from build123d import *

# Parameters (mm, degrees)
F0_W           = 9.5
F0_H           = 60
F1_DEPTH       = 4.5
F4_D           = 3.1
F4_CBORE_D     = 5.9
F4_CBORE_DEPTH = 2.2
F5_DEPTH       = 25
F6_SIZE        = 5
F7_R           = 3


with BuildPart() as f1:
    # F0 (on Top) → F1 (new body)
    with BuildSketch(Plane.XY):
        with Locations((4.75, 30)):
            Rectangle(F0_W, F0_H)
    extrude(amount=F1_DEPTH)

    # F4 (through all)
    with Locations(Plane.XY.offset(4.5)):
        with Locations((5.4, 36.5), (5.4, 5.5)):
            CounterBoreHole(F4_D / 2, F4_CBORE_D / 2, F4_CBORE_DEPTH)

    # F3 (on face) → F5 (cut)
    with BuildSketch(Plane.XY.offset(4.5)):
        with BuildLine():
            Line((6.25, 57.5), (3.25, 57.5))
            ThreePointArc((3.25, 57.5), (2.542893, 57.207107), (2.25, 56.5))
            Line((2.25, 56.5), (2.25, 44))
            ThreePointArc((2.25, 44), (2.542893, 43.292893), (3.25, 43))
            Line((3.25, 43), (6.25, 43))
            ThreePointArc((6.25, 43), (6.957107, 43.292893), (7.25, 44))
            Line((7.25, 44), (7.25, 56.5))
            ThreePointArc((7.25, 56.5), (6.957107, 57.207107), (6.25, 57.5))
        make_face()
    extrude(amount=-F5_DEPTH, mode=Mode.SUBTRACT)

    # F6
    f6_edges = [f1.edges().sort_by_distance(p)[0] for p in [
        (0, 0, 2.25),
    ]]
    chamfer(f6_edges, length=F6_SIZE)

    # F7
    f7_edges = [f1.edges().sort_by_distance(p)[0] for p in [
        (0, 60, 2.25),
        (9.5, 60, 2.25),
    ]]
    fillet(f7_edges, radius=F7_R)


solid = f1.part
Model file for the job. Use its own axes, mm. A direction names the side the tool comes from. Give positions to 0.01 mm unless a question says otherwise; leave off trailing zeros. Write each loop counter-clockwise with the first axis right and the second up, starting at its lowest first coordinate (ties: lowest second). Pieces come first, ordered by that corner, then holes. Notation, with made-up numbers: M 21,-27 L 33,-27 A5 ccw 33,-18 Z; hole C 50,-39 d11. An arc over 180 degrees is marked long. One line per item, written item: value. Start each with the question number.
Q1. Saw through at A-A, the plane z = 1. Write the cut outline in (x, y).
Q2. 3-axis set-ups, long thin cutter, end or side, ignore diameter. For faces 1 (the flat face through (5, 24, 0)), 2 (the flat face through (7, 4, 2.3)), 3 (the flat face through (5, 43, 2)): which of +Z, -Z, +X, -X, +Y, -Y reach the whole face in a straight line?
Q3. Probe probe 1 along Y at (x, z) = (5.4, 3.3); probe 2 along Y at (x, z) = (5.4, 1.4); probe 3 along Y at (x, z) = (7.5, 4.35). List the from-to ranges inside material, lowest first. Write a range as [from, to].
Q4. Drop flat-ended pins along their axis: pin 1 Ø3.5 at (x, y) = (5.4, 36.5) entering from +Z; pin 2 Ø2 at (x, z) = (8.5, 2) entering from +Y. Give the stop position or say it passes through.
Q5. Saw through at D-D, the plane y = 4.5. Write the cut outline in (x, z).
Q6. Saw through at C-C, the plane z = 3.9. Write the cut outline in (x, y).
Q7. Saw through at B-B, the plane y = 36.5. Write the cut outline in (x, z).
Q8. Two-plate mould, pull along X, no slides. Class faces 4 (the flat face through (5, 24, 4.5)), 5 (the cylindrical face through (6.949, 43.285, 2.282)), 6 (the cylindrical face through (2.535, 43.301, 2.282)), 7 (the cylindrical face through (8.6, 59.14, 2.28)): +X half, -X half, draft (parallel to the pull), parting line (faces both ways), or undercut.
Output values:
1. outline: M 0,5 L 5,0 L 9.5,0 L 9.5,57 A3 ccw 6.5,60 L 3,60 A3 ccw 0,57 Z; hole M 2.25,44 A1 ccw 3.25,43 L 6.25,43 A1 ccw 7.25,44 L 7.25,56.5 A1 ccw 6.25,57.5 L 3.25,57.5 A1 ccw 2.25,56.5 Z; hole C 5.4,5.5 d3.1; hole C 5.4,36.5 d3.1
2. face 1: -Z, +X, -X, +Y, -Y
2. face 2: +Z
2. face 3: +Z, -Z
3. probe 1: y = [0, 2.55], [8.45, 33.55], [39.45, 43], [57.5, 60]
3. probe 2: y = [0, 3.95], [7.05, 34.95], [38.05, 43], [57.5, 60]
3. probe 3: y = [0, 3.43], [7.57, 34.43], [38.57, 59.83]
4. pin 1: stops at z = 2.3
4. pin 2: stops at y = 59.83
5. outline: M 0.5,0 L 4.22,0 L 4.22,2.3 L 2.62,2.3 L 2.62,4.5 L 0.5,4.5 Z; M 6.58,0 L 9.5,0 L 9.5,4.5 L 8.18,4.5 L 8.18,2.3 L 6.58,2.3 Z
6. outline: M 0,5 L 5,0 L 9.5,0 L 9.5,57 A3 ccw 6.5,60 L 3,60 A3 ccw 0,57 Z; hole M 2.25,44 A1 ccw 3.25,43 L 6.25,43 A1 ccw 7.25,44 L 7.25,56.5 A1 ccw 6.25,57.5 L 3.25,57.5 A1 ccw 2.25,56.5 Z; hole C 5.4,5.5 d5.9; hole C 5.4,36.5 d5.9
7. outline: M 0,0 L 3.85,0 L 3.85,2.3 L 2.45,2.3 L 2.45,4.5 L 0,4.5 Z; M 6.95,0 L 9.5,0 L 9.5,4.5 L 8.35,4.5 L 8.35,2.3 L 6.95,2.3 Z
8. face 4: draft
8. face 5: undercut
8. face 6: undercut
8. face 7: +X half
